Check sheet for the modelled part. Datum: model origin and axes. Units: mm. Face numbers are marked on the shaded views. A direction names the side the tool comes from. Coordinates: 2 decimals unless noted, no trailing zeros. Write each loop counter-clockwise with the first axis right and the second up, starting at its lowest first coordinate (ties: lowest second). Pieces come first, ordered by that corner, then holes. Notation, with made-up numbers: (78.5, 55.25) - (120.5, 55.25) arc R9 ccw to (120.5, 59.25) - close; hole circle Ø9 at (-21.5, 23.5). An arc over 180 degrees is marked (long way). Use one line per item in the form item = value. Start each with the question number.
1. Go/stop test with flat-tipped pins: pin 1 Ø6 at (y, z) = (-17, 6.5) entering from +X; pin 2 Ø2.5 at (x, y) = (-36, 0) entering from +Z; pin 3 Ø6 at (y, z) = (-25.5, 4) entering from +X; pin 4 Ø4 at (x, y) = (-6.5, 13.5) entering from +Z. Record where each tip stops, or that it passes through.
2. Scan lines: line 1 along Y through (x, z) = (-36, 1.1); line 2 along Y through (x, z) = (6.5, 2.5); line 3 along X through (y, z) = (14.5, 1). Record each from-to range of solid material in increasing order.
3. Cross-section at D-D on x = -27. Record the boundary of the cut face in (y, z), then the cut area to 3 significant figures.
4. Cross-section at C-C on y = 12.5. Record the boundary of the cut face in (x, z), then the cut area to 3 significant figures.
5. Cross-section at A-A on x = 36. Record the boundary of the cut face in (y, z), then the cut area to 3 significant figures.
6. Tool access check on the marked faces 1, 2 and 3. Record the directions out of +Z, -Z, +X, -X, +Y, -Y that give a thin tool (end or side, any length) a straight path to the whole face; none if there is none.
7. Cross-section at B-B on y = -15.5. Record the boundary of the cut face in (x, z), then the cut area to 3 significant figures.
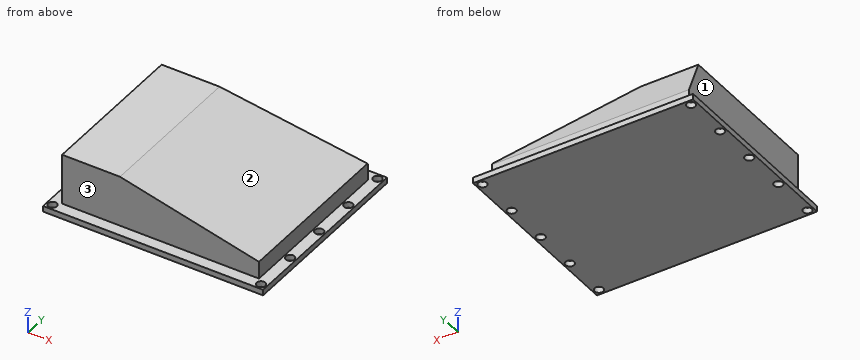
```python
from build123d import *

# Parameters (mm, degrees)
F0_W     = 76
F0_H     = 66
F1_DEPTH = 2
F2_W     = 68
F2_H     = 58
F3_DEPTH = 17.5
F5_DEPTH = 75
F6_SIZE2 = 12
F6_SIZE  = 5
F7_R     = 1.5
F8_DEPTH = 25


with BuildPart() as f1:
    # F0 (on Top) → F1 (new body)
    with BuildSketch(Plane.XY):
        Rectangle(F0_W, F0_H)
    extrude(amount=F1_DEPTH)

    # F2 (on face) → F3 (join)
    with BuildSketch(Plane.XY.offset(2)):
        Rectangle(F2_W, F2_H)
    extrude(amount=F3_DEPTH)

    # F4 (on face) → F5 (cut)
    with BuildSketch(Plane(origin=(0, 29, 0), x_dir=(-1, 0, 0), z_dir=(0, 1, 0))):
        Polygon((14, 19.5), (-34, 19.5), (-34, 8), align=None)
    extrude(amount=-F5_DEPTH, mode=Mode.SUBTRACT)

    # F6
    f6_edges = [f1.edges().sort_by_distance(p)[0] for p in [
        (-24, 29, 19.5),
    ]]
    f6_side = f1.faces().sort_by_distance((-24, 0, 19.5))[0]
    chamfer(f6_edges, length=F6_SIZE, length2=F6_SIZE2, reference=f6_side)

    # F7 (on face) → F8 (cut)
    with BuildSketch(Plane.XY.offset(2)):
        with Locations((-36, 31)):
            Circle(F7_R)
        with Locations((-36, 0)):
            Circle(F7_R)
        with Locations((-36, -31)):
            Circle(F7_R)
        with Locations((36, 31)):
            Circle(F7_R)
        with Locations((36, 0)):
            Circle(F7_R)
        with Locations((36, -31)):
            Circle(F7_R)
        with Locations((-36, 15.5)):
            Circle(F7_R)
        with Locations((-36, -15.5)):
            Circle(F7_R)
        with Locations((36, 15.5)):
            Circle(F7_R)
        with Locations((36, -15.5)):
            Circle(F7_R)
    extrude(amount=-F8_DEPTH, mode=Mode.SUBTRACT)


solid = f1.part
```
Final values:
q1.pin_1 = 34
q1.pin_2 = through
q1.pin_3 = 38
q1.pin_4 = 18.18
q2.line_1 = -33 to -32.5, -29.5 to -17, -14 to -1.5, 1.5 to 14, 17 to 29.5, 32.5 to 33
q2.line_2 = -29 to 29
q2.line_3 = -38 to -37.12, -34.88 to 34.88, 37.12 to 38
q3.outline = (-33, 0) - (33, 0) - (33, 2) - (29, 2) - (29, 7.5) - (24, 19.5) - (-29, 19.5) - (-29, 2) - (-33, 2) - close
q3.area = 1,120 mm²
q4.outline = (-38, 0) - (38, 0) - (38, 2) - (34, 2) - (34, 8) - (-14, 19.5) - (-34, 19.5) - (-34, 2) - (-38, 2) - close
q4.area = 1,070 mm²
q5.outline = (-33, 0) - (-32.5, 0) - (-32.5, 2) - (-33, 2) - close; (-29.5, 0) - (-17, 0) - (-17, 2) - (-29.5, 2) - close; (-14, 0) - (-1.5, 0) - (-1.5, 2) - (-14, 2) - close; (1.5, 0) - (14, 0) - (14, 2) - (1.5, 2) - close; (17, 0) - (29.5, 0) - (29.5, 2) - (17, 2) - close; (32.5, 0) - (33, 0) - (33, 2) - (32.5, 2) - close
q5.area = 102 mm²
q6.face_1 = +Z, -X, +Y, -Y
q6.face_2 = +Z, +X, +Y, -Y
q6.face_3 = +Z, +X, -X, -Y
q7.outline = (-38, 0) - (-37.5, 0) - (-37.5, 2) - (-38, 2) - close; (-34.5, 0) - (34.5, 0) - (34.5, 2) - (34, 2) - (34, 8) - (-14, 19.5) - (-34, 19.5) - (-34, 2) - (-34.5, 2) - close; (37.5, 0) - (38, 0) - (38, 2) - (37.5, 2) - close
q7.area = 1,050 mm²
